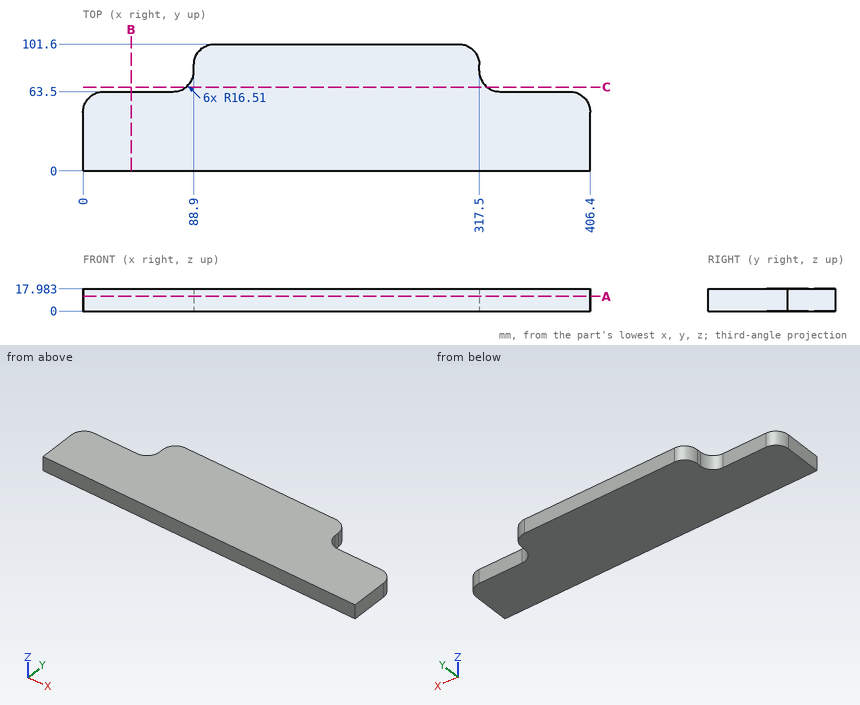
The figure shows three views and two pictorial views of one solid part (mm, origin at its lowest corner). Answer the questions. Coordinates: 2 decimals unless noted, no trailing zeros. Loops run counter-clockwise (first coordinate to the right, second up) from the corner with the lowest first, then second, coordinate; pieces in that order, holes last. Notation, with made-up numbers: (-24, -39) - (18, -39) arc R23 ccw to (18, -28) - close; hole circle Ø3 at (42, -14.75). An arc over 180 degrees is marked (long way). Write item = value, one per line.
1) Section B-B (x = 38.5) is taken. Determine the outline of the cut face in (y, z), plus the area to 3 significant figures.
Responses:
outline = (0, 0) - (63.5, 0) - (63.5, 17.98) - (0, 17.98) - close
area = 1,140 mm^2
2) Section A-A (z = 12) is taken. Determine the outline of the cut face in (x, y), plus the area to 3 significant figures.
Responses:
outline = (0, 0) - (406.4, 0) - (406.4, 46.99) arc R16.51 ccw to (389.89, 63.5) - (334.01, 63.5) arc R16.51 cw to (317.5, 80.01) - (317.5, 85.09) arc R16.51 ccw to (300.99, 101.6) - (105.41, 101.6) arc R16.51 ccw to (88.9, 85.09) - (88.9, 80.01) arc R16.51 cw to (72.39, 63.5) - (16.51, 63.5) arc R16.51 ccw to (0, 46.99) - close
area = 34,400 mm^2
3) Section C-C (y = 67) is taken. Determine the outline of the cut face in (x, z) (1 decimal).
Responses:
outline = (82.6, 0) - (323.8, 0) - (323.8, 18) - (82.6, 18) - close
4) Each of these flat-tipped pins is pushed along its axis until it touches: P1, Ø3, axis at y = 62.5, z = 3, coming from the -X side (1 decimal); P2, Ø9, axis at x = 58, z = 13, coming from the +Y side; P3, Ø8, axis at y = 82.5, z = 14, coming from the +X side. Where does it stop, or does it pass through?
Responses:
P1 = 7.8
P2 = 63.5
P3 = 317.57
5) Find the intervals of material crossed by line 1 along X through (y, z) = (81.5, 9.5); line 2 along X through (y, z) = (48.5, 16.5); line 3 along Y through (x, z) = (309, 3.5), in increasing order.
Responses:
line_1 = 88.9 to 317.5
line_2 = 0.07 to 406.33
line_3 = 0 to 99.53
